The listing builds one solid part. Answer for the finished solid, in the listing's coordinates (mm). Face numbers are marked on the shaded views. A direction names the side the tool comes from. Round coordinates to 2 decimals unless told otherwise and drop trailing zeros. Write each loop counter-clockwise with the first axis right and the second up, starting at its lowest first coordinate (ties: lowest second). Pieces come first, ordered by that corner, then holes. Notation, with made-up numbers: M -38.5,3.5 L -23.5,3.5 A27 cw -23.5,23.5 Z; hole C -29,16 d11. An arc over 180 degrees is marked long. Write each question's results on one line, items separated by ' | '.
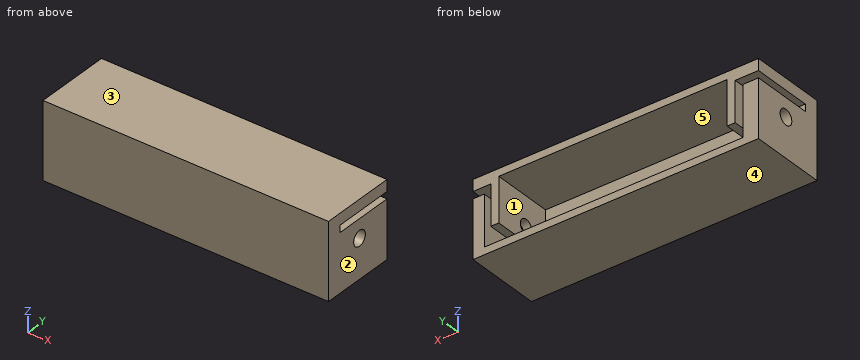
from build123d import *

# Parameters (mm, degrees)
SKETCH1_W           = 75
SKETCH1_H           = 20
BOSS_EXTRUDE1_DEPTH = 20
CUT_EXTRUDE2_DEPTH  = 16
SKETCH3_R           = 2
CUT_EXTRUDE3_DEPTH  = 96


with BuildPart() as part:
    # Sketch1 → Boss-Extrude1 (new body)
    with BuildSketch(Plane.XY):
        with Locations((-0.726872247, 21.927312775)):
            Rectangle(SKETCH1_W, SKETCH1_H)
    extrude(amount=BOSS_EXTRUDE1_DEPTH)

    # Sketch2 → Cut-Extrude2 (cut)
    with BuildSketch(Plane(origin=(0, 31.927312775, 0), x_dir=(1, 0, 0), z_dir=(0, 1, 0))):
        Polygon((36.773127753, -16.997338724), (36.773127753, -15.156017778), (34.105822873, -15.156017778), (33.814685074, -15.156017778), (33.814685074, -4.376760328), (33.814685074, -1.902190301), (32.105822873, -1.902190301), (-32.105822873, -1.902190301), (-34.105822873, -1.902190301), (-34.105822873, -4.376760328), (-34.105822873, -15.156017778), (-38.226872247, -15.156017778), (-38.226872247, -16.997338724), (-32.105822873, -16.997338724), (-32.105822873, -6.427465258), (-30, -6.427465258), (-30, -18.05964209), (30, -18.05964209), (30, -6.427465258), (32.105822873, -6.427465258), (32.105822873, -16.997338724), align=None)
    extrude(amount=-CUT_EXTRUDE2_DEPTH, mode=Mode.SUBTRACT)

    # Sketch3 → Cut-Extrude3 (cut)
    with BuildSketch(Plane(origin=(36.773127753, 0, 0), x_dir=(0, 0, -1), z_dir=(1, 0, 0))):
        with Locations(Location((-10.245692038, 22.537083277, 0), (0, 0, 90))):
            Circle(SKETCH3_R)
    extrude(amount=-CUT_EXTRUDE3_DEPTH, mode=Mode.SUBTRACT)


solid = part.part
1) A tool of negligible diameter and unlimited length cuts with its end or side. For the marked faces 4 and 5, from which of +Z, -Z, +X, -X, +Y, -Y can it reach the whole face along a straight path? Write none if from no direction.
Return value:
face 4: -Z, +X, -X, +Y, -Y | face 5: +Y
2) Section A-A (y = 30) is taken. Determine the outline of the cut face in (x, z), then the cut area to 3 significant figures.
Return value:
outline: M -38.23,0 L 36.77,0 L 36.77,15.16 L 33.81,15.16 L 33.81,1.9 L -34.11,1.9 L -34.11,15.16 L -38.23,15.16 Z; M -38.23,17 L -32.11,17 L -32.11,6.43 L -30,6.43 L -30,18.06 L 30,18.06 L 30,6.43 L 32.11,6.43 L 32.11,17 L 36.77,17 L 36.77,20 L -38.23,20 Z | area: 442 mm²
3) Section D-D (z = 16) is taken. Determine the outline of the cut face in (x, y).
Return value:
outline: M -38.23,11.93 L 36.77,11.93 L 36.77,15.93 L 32.11,15.93 L 32.11,31.93 L 30,31.93 L 30,15.93 L -30,15.93 L -30,31.93 L -32.11,31.93 L -32.11,15.93 L -38.23,15.93 Z
4) This flat-tipped pin is pushed along its axis until it touches: pin 1 (3 mm diameter, centred on x = 23.5, z = 8, fed in from +Y). Where does it stop, or does it pass through?
Return value:
pin 1: y = 15.93
5) The mould has two halves that part along X. Classify the marked faces 1, 2 and 3: +X half, -X half, draft (parallel to the pull), parting line (faces both ways), or undercut.
Return value:
face 1: undercut | face 2: +X half | face 3: draft
6) Section C-C (x = -3) is taken. Determine the outline of the cut face in (y, z), then the cut area to 3 significant figures.
Return value:
outline: M 11.93,0 L 31.93,0 L 31.93,1.9 L 15.93,1.9 L 15.93,18.06 L 31.93,18.06 L 31.93,20 L 11.93,20 Z | area: 141 mm²
7) Find the intervals of material crossed by line 1 (Z direction, x = -14, y = 26.5); line 2 (X direction, y = 24.25, z = 4.75); line 3 (X direction, y = 24.25, z = 18), in increasing order.
Return value:
line 1: 0 to 1.9, 18.06 to 20 | line 2: -38.23 to -34.11, 33.81 to 36.77 | line 3: -38.23 to -30, 30 to 36.77
8) Section B-B (z = 3.25) is taken. Determine the outline of the cut face in (x, y), then the cut area to 3 significant figures.
Return value:
outline: M -38.23,11.93 L 36.77,11.93 L 36.77,31.93 L 33.81,31.93 L 33.81,15.93 L -34.11,15.93 L -34.11,31.93 L -38.23,31.93 Z | area: 413 mm²
